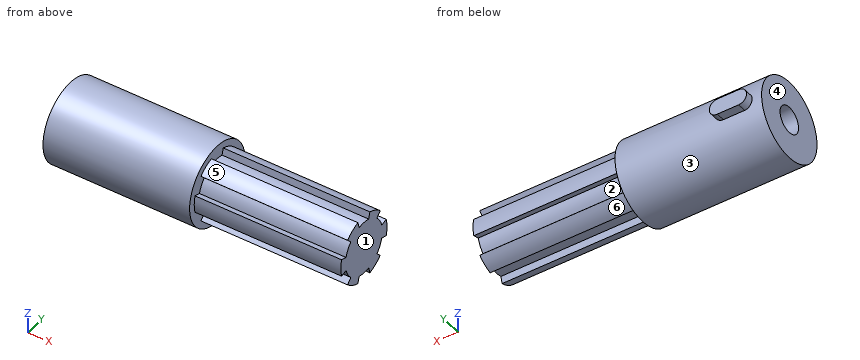
from build123d import *

# Parameters (mm, degrees)
SKETCH_1_R          = 15
EXTRUDE_1_DEPTH     = 55
SKETCH_2_R          = 10
EXTRUDE_2_DEPTH     = 55
SKETCH_3_R          = 5
CUT_EXTRUDE_1_DEPTH = 25
EXTRUDE_START       = 10
EXTRUDE_3_DEPTH     = 8


with BuildPart() as part:
    # 草图1 → 凸台-拉伸1 (new body)
    with BuildSketch(Plane(origin=(0, 0, 0), x_dir=(0, 0, -1), z_dir=(1, 0, 0))):
        Circle(SKETCH_1_R)
    extrude(amount=EXTRUDE_1_DEPTH)

    # 草图2 → 凸台-拉伸2 (add)
    with BuildSketch(Plane(origin=(55, 0, 0), x_dir=(0, 0, -1), z_dir=(1, 0, 0))):
        with BuildLine():
            ThreePointArc((-9.659258263, 2.588190451), (-8.660254038, 5), (-7.071067812, 7.071067812))
            Line((-7.071067812, 7.071067812), (-8.825622579, 8.852027231))
            ThreePointArc((-8.825622579, 8.852027231), (-10.8206468, 6.258083), (-12.074072829, 3.235238064))
            Line((-12.074072829, 3.235238064), (-9.659258263, 2.588190451))
        make_face()
        Circle(SKETCH_2_R)
        with BuildLine():
            ThreePointArc((3.253269167, 12.069226973), (0.009335457, 12.499996514), (-3.235238064, 12.074072829))
            Line((-3.235238064, 12.074072829), (-2.588190451, 9.659258263))
            ThreePointArc((-2.588190451, 9.659258263), (0, 10), (2.588190451, 9.659258263))
            Line((2.588190451, 9.659258263), (3.253269167, 12.069226973))
        make_face()
        with BuildLine():
            Line((8.838834765, 8.838834765), (7.071067812, 7.071067812))
            ThreePointArc((7.071067812, 7.071067812), (8.660254038, 5), (9.659258263, 2.588190451))
            Line((9.659258263, 2.588190451), (12.078891746, 3.217199742))
            ThreePointArc((12.078891746, 3.217199742), (10.829982257, 6.241913514), (8.838834765, 8.838834765))
        make_face()
        with BuildLine():
            Line((12.074072829, -3.235238064), (9.659258263, -2.588190451))
            ThreePointArc((9.659258263, -2.588190451), (8.660254038, -5), (7.071067812, -7.071067812))
            Line((7.071067812, -7.071067812), (8.825622579, -8.852027231))
            ThreePointArc((8.825622579, -8.852027231), (10.8206468, -6.258083), (12.074072829, -3.235238064))
        make_face()
        with BuildLine():
            ThreePointArc((2.588190451, -9.659258263), (0, -10), (-2.588190451, -9.659258263))
            Line((-2.588190451, -9.659258263), (-3.253269167, -12.069226973))
            ThreePointArc((-3.253269167, -12.069226973), (-0.009335457, -12.499996514), (3.235238064, -12.074072829))
            Line((3.235238064, -12.074072829), (2.588190451, -9.659258263))
        make_face()
        with BuildLine():
            ThreePointArc((-7.071067812, -7.071067812), (-8.660254038, -5), (-9.659258263, -2.588190451))
            Line((-9.659258263, -2.588190451), (-12.078891746, -3.217199742))
            ThreePointArc((-12.078891746, -3.217199742), (-10.829982257, -6.241913514), (-8.838834765, -8.838834765))
            Line((-8.838834765, -8.838834765), (-7.071067812, -7.071067812))
        make_face()
    extrude(amount=EXTRUDE_2_DEPTH)

    # 草图3 → 切除-拉伸1 (cut)
    with BuildSketch(Plane.ZY):
        Circle(SKETCH_3_R)
    extrude(amount=-CUT_EXTRUDE_1_DEPTH, mode=Mode.SUBTRACT)

    # 草图4 → 凸台-拉伸3 (add)
    with BuildSketch(Plane(origin=(0, 0, 0), x_dir=(1, 0, 0), z_dir=(0, 1, 0)).offset(EXTRUDE_START)):
        with BuildLine():
            Line((6.545306006, 3), (14.545306006, 3))
            ThreePointArc((14.545306006, 3), (17.545306006, 0), (14.545306006, -3))
            Line((14.545306006, -3), (6.545306006, -3))
            ThreePointArc((6.545306006, -3), (3.545306006, 0), (6.545306006, 3))
        make_face()
    extrude(amount=EXTRUDE_3_DEPTH)


solid = part.part
Read the model definition and answer for the solid it produces. Units are mm, in the model's axes. Face numbers are marked on the shaded views. A direction names the side the tool comes from. Coordinates: 2 decimals unless noted, no trailing zeros. Loops run counter-clockwise (first coordinate to the right, second up) from the corner with the lowest first, then second, coordinate; pieces in that order, holes last.
Q1. The mould has two halves that part along Z. Classify the marked faces 1, 2 and 3: +Z half, -Z half, draft (parallel to the pull), parting line (faces both ways), or undercut.
Q2. Each of these flat-tipped pins is pushed along its axis until it touches: pin 1 Ø3 at (x, y) = (34.5, 13) entering from -Z; pin 2 Ø12 at (x, y) = (82, 10) entering from -Z; pin 3 Ø8 at (y, z) = (-1.5, 1.5) entering from -X; pin 4 Ø10 at (x, z) = (81.5, 7) entering from -Y. Where does it stop, or does it pass through?
Q3. The part is cut by section B-B on x = 74. Write down the section's boundary in (y, z), and give its area (3 significant figures).
Q4. Consider probe 1 along Y at (x, z) = (18, 0); probe 2 along Y at (x, z) = (5, 0); probe 3 along X at (y, z) = (0, -0.5). Determine where each line is inside the solid, lowest interval first.
Q5. The part is cut by section A-A on y = 0. Write down the section's boundary in (x, z), and give its area (3 significant figures).
Q6. Which of the six approach directions +Z, -Z, +X, -X, +Y, -Y give full straight-line access (tool end or side, diameter ignored) to the marked faces 4, 5 and 6?
Q7. The part is cut by section D-D on x = 21.5. Write down the section's boundary in (y, z), and give its area (3 significant figures).
Q8. The part is cut by section C-C on z = 0. Write down the section's boundary in (x, y), and give its area (3 significant figures).
Results below:
1. face 1: draft
1. face 2: undercut
1. face 3: parting line
2. pin 1: stops at z = -9.63
2. pin 2: stops at z = -11.84
2. pin 3: stops at x = 0
2. pin 4: stops at y = -12.34
3. outline: (-12.07, -3.24) - (-9.66, -2.59) arc R10 ccw to (-7.07, -7.07) - (-8.85, -8.83) arc R12.5 ccw to (-3.24, -12.07) - (-2.59, -9.66) arc R10 ccw to (2.59, -9.66) - (3.22, -12.08) arc R12.5 ccw to (8.84, -8.84) - (7.07, -7.07) arc R10 ccw to (9.66, -2.59) - (12.07, -3.25) arc R12.5 ccw to (12.07, 3.24) - (9.66, 2.59) arc R10 ccw to (7.07, 7.07) - (8.85, 8.83) arc R12.5 ccw to (3.24, 12.07) - (2.59, 9.66) arc R10 ccw to (-2.59, 9.66) - (-3.22, 12.08) arc R12.5 ccw to (-8.84, 8.84) - (-7.07, 7.07) arc R10 ccw to (-9.66, 2.59) - (-12.07, 3.25) arc R12.5 ccw to start
3. area: 403 mm2
4. probe 1: y = -15 to -5, 5 to 15
4. probe 2: y = -15 to -5, 5 to 18
4. probe 3: x = 25 to 110
5. outline: (0, -15) - (55, -15) - (55, -10) - (110, -10) - (110, 10) - (55, 10) - (55, 15) - (0, 15) - (0, 5) - (25, 5) - (25, -5) - (0, -5) - close
5. area: 2,500 mm2
6. face 4: +Z, -Z, -X, +Y, -Y
6. face 5: +Z, +X, -Y
6. face 6: -Z, +X, +Y
7. outline: circle Ø30 at (0, 0); hole circle Ø10 at (0, 0)
7. area: 628 mm2
8. outline: (0, -15) - (55, -15) - (55, -12.5) - (110, -12.5) - (110, 12.5) - (55, 12.5) - (55, 15) - (17.55, 15) - (17.55, 18) - (3.55, 18) - (3.55, 15) - (0, 15) - (0, 5) - (25, 5) - (25, -5) - (0, -5) - close
8. area: 2,820 mm2
